Read the model definition and answer for the solid it produces. Units are mm, in the model's axes. A direction names the side the tool comes from. Round coordinates to 2 decimals unless told otherwise and drop trailing zeros. Loops run counter-clockwise (first coordinate to the right, second up) from the corner with the lowest first, then second, coordinate; pieces in that order, holes last. Notation, with made-up numbers: (76, 3.5) - (119, 3.5) arc R28 cw to (119, 35.5) - close; hole circle Ø5 at (32, -31). An arc over 180 degrees is marked (long way). Use one line per item in the form item = value. Start each with the question number.
```python
from build123d import *

# Parameters (mm, degrees)
SKETCH_1_R      = 1.6
SKETCH_1_R_2    = 5.5
EXTRUDE_2_DEPTH = 2.5
SKETCH_2_R      = 1.6
EXTRUDE_3_DEPTH = 2.5


with BuildPart() as part:
    # 草图1 → 凸台-拉伸2 (new body)
    with BuildSketch(Plane.XY):
        with BuildLine():
            Line((-1.519577757, 8.363066629), (22.821226146, 12.785815586))
            ThreePointArc((22.821226146, 12.785815586), (23.640790975, 12.569640788), (24, 11.801925394))
            Line((24, 11.801925394), (24, -11.801925394))
            ThreePointArc((24, -11.801925394), (23.640790975, -12.569640788), (22.821226146, -12.785815586))
            Line((22.821226146, -12.785815586), (-1.519577757, -8.363066629))
            ThreePointArc((-1.519577757, -8.363066629), (-8.5, 0), (-1.519577757, 8.363066629))
        make_face()
        with Locations((20, 8.75)):
            Circle(SKETCH_1_R, mode=Mode.SUBTRACT)
        with Locations((20, -8.75)):
            Circle(SKETCH_1_R, mode=Mode.SUBTRACT)
        Circle(SKETCH_1_R_2, mode=Mode.SUBTRACT)
    extrude(amount=EXTRUDE_2_DEPTH)

    # 草图2 → 凸台-拉伸3 (add)
    with BuildSketch(Plane.XY.offset(2.5)):
        with BuildLine():
            Line((-1.519577757, -8.363066629), (22.821226146, -12.785815586))
            ThreePointArc((22.821226146, -12.785815586), (23.640790975, -12.569640788), (24, -11.801925394))
            Line((24, -11.801925394), (24, 11.801925394))
            ThreePointArc((24, 11.801925394), (23.640790975, 12.569640788), (22.821226146, 12.785815586))
            Line((22.821226146, 12.785815586), (-1.519577757, 8.363066629))
            ThreePointArc((-1.519577757, 8.363066629), (-8.5, 0), (-1.519577757, -8.363066629))
        make_face()
        with Locations((20, -8.75)):
            Circle(SKETCH_2_R, mode=Mode.SUBTRACT)
        with Locations((20, 8.75)):
            Circle(SKETCH_2_R, mode=Mode.SUBTRACT)
    extrude(amount=EXTRUDE_3_DEPTH)


solid = part.part
```
1) A cutting plane is placed at A-A on x = 20. Write down the section's boundary in (y, z).
2) For faces 1 (the flat face through (0, 0, 2.5)), 2 (the cylindrical face through (-8.5, 0.17, 2.46)), determine the directions among +Z, -Z, +X, -X, +Y, -Y from which every point of the face is accessible in a straight line to the end or side of a thin tool.
3) Flat-ended cylindrical pins translate along their axes: pin 1 (1.5 mm diameter, centred on y = -5.5, z = 2.5, fed in from -X); pin 2 (3 mm diameter, centred on x = 11.5, z = 2, fed in from +Y); pin 3 (2 mm diameter, centred on y = 5, z = 3, fed in from -X). Find the tip coordinate at first contact, or state that the pin passes through.
4) Determine the mould class of faces 3 (the flat face through (11, 0, 5)), 4 (the cylindrical face through (19, -10, 2)), 5 (the cylindrical face through (-1.19, -5.37, 1.23)), 6 (the flat face through (10.48, -10.543, 2.465)) for opening direction X: +X half, -X half, draft (parallel to the pull), parting line (faces both ways), or undercut.
5) A cutting plane is placed at D-D on y = 4. Write down the section's boundary in (x, z), plus the area to 3 significant figures.
6) Straight lines are drawn through the part: line 1 (Y direction, x = 20, z = 2.8); line 2 (X direction, y = -4.75, z = 2.2); line 3 (X direction, y = -0.25, z = 3.75). For each, find the intervals that lie inside material, in ascending order. Write a range as from..to.
7) A cutting plane is placed at C-C on y = -9.25. Write down the section's boundary in (x, z).
8) A cutting plane is placed at B-B on z = 0.35. Write down the section's boundary in (x, y).
Checks:
q1.outline = (-12.27, 0) - (-10.35, 0) - (-10.35, 5) - (-12.27, 5) - close; (-7.15, 0) - (7.15, 0) - (7.15, 5) - (-7.15, 5) - close; (10.35, 0) - (12.27, 0) - (12.27, 5) - (10.35, 5) - close
q2.face_1 = -Z
q2.face_2 = +Z, -Z, -X
q3.pin_1 = -7.05
q3.pin_2 = 11
q3.pin_3 = -7.5
q4.face_3 = draft
q4.face_4 = undercut
q4.face_5 = undercut
q4.face_6 = -X half
q5.outline = (-7.5, 0) - (-3.77, 0) - (-3.77, 2.5) - (3.77, 2.5) - (3.77, 0) - (24, 0) - (24, 5) - (-7.5, 5) - close
q5.area = 139 mm²
q6.line_1 = -12.27..-10.35, -7.15..7.15, 10.35..12.27
q6.line_2 = -7.05..-2.77, 2.77..24
q6.line_3 = -8.5..24
q7.outline = (3.36, 0) - (18.48, 0) - (18.48, 5) - (3.36, 5) - close; (21.52, 0) - (24, 0) - (24, 5) - (21.52, 5) - close
q8.outline = (-1.52, -8.36) - (22.82, -12.79) arc R1 ccw to (24, -11.8) - (24, 11.8) arc R1 ccw to (22.82, 12.79) - (-1.52, 8.36) arc R8.5 ccw to start; hole circle Ø11 at (0, 0); hole circle Ø3.2 at (20, -8.75); hole circle Ø3.2 at (20, 8.75)
